Model file for the job. Use its own axes, mm. A direction names the side the tool comes from. Give positions to 0.01 mm unless a question says otherwise; leave off trailing zeros. Write each loop counter-clockwise with the first axis right and the second up, starting at its lowest first coordinate (ties: lowest second). Pieces come first, ordered by that corner, then holes.
```python
from build123d import *

# Parameters (mm, degrees)
SKETCH1_W                                         = 100
SKETCH1_H                                         = 20
BOSS_EXTRUDE1_DEPTH                               = 3
SKETCH2_R                                         = 4
SKETCH2_R_2                                       = 3
SKETCH2_R_3                                       = 5
BOSS_EXTRUDE2_DEPTH                               = 9
CHAMFER1_SIZE                                     = 3
CSK_FOR_6_FLAT_HEAD_MACHINE_SCREW_100_D           = 3.7973
CSK_FOR_6_FLAT_HEAD_MACHINE_SCREW_100_CSINK_D     = 7.0866
CSK_FOR_6_FLAT_HEAD_MACHINE_SCREW_100_CSINK_ANGLE = 100
CSK_FOR_6_FLAT_HEAD_MACHINE_SCREW_2_D             = 3.7973
CSK_FOR_6_FLAT_HEAD_MACHINE_SCREW_2_CSINK_D       = 7.0866
CSK_FOR_6_FLAT_HEAD_MACHINE_SCREW_2_CSINK_ANGLE   = 100
CSK_FOR_6_FLAT_HEAD_MACHINE_SCREW_3_D             = 3.7973
CSK_FOR_6_FLAT_HEAD_MACHINE_SCREW_3_CSINK_D       = 7.0866
CSK_FOR_6_FLAT_HEAD_MACHINE_SCREW_3_CSINK_ANGLE   = 100
CHAMFER2_SIZE                                     = 3
CHAMFER3_SIZE                                     = 3
SKETCH14_R                                        = 3
SKETCH14_R_2                                      = 4
SKETCH14_R_3                                      = 5
BOSS_EXTRUDE3_DEPTH                               = 3
CHAMFER4_SIZE                                     = 3
LPATTERN1_COUNT                                   = 3
LPATTERN1_PITCH                                   = 15
CHAMFER5_SIZE                                     = 7


with BuildPart() as part:
    # Sketch1 → Boss-Extrude1 (new body)
    with BuildSketch(Plane(origin=(0, 0, 0), x_dir=(1, 0, 0), z_dir=(0, 1, 0))):
        Rectangle(SKETCH1_W, SKETCH1_H)
    extrude(amount=BOSS_EXTRUDE1_DEPTH)

    # Sketch2 → Boss-Extrude2 (add)
    with BuildSketch(Plane(origin=(0, 3, 0), x_dir=(1, 0, 0), z_dir=(0, 1, 0))):
        with Locations(Location((-25, 0, 0), (0, 0, 90))):
            Circle(SKETCH2_R)
        with Locations(Location((-40, 0, 0), (0, 0, 90))):
            Circle(SKETCH2_R_2)
        with Locations(Location((-10, 0, 0), (0, 0, 90))):
            Circle(SKETCH2_R_3)
    extrude(amount=BOSS_EXTRUDE2_DEPTH)

    # Chamfer1
    chamfer1_edges = [part.edges().sort_by_distance(p)[0] for p in [
        (-40, 3, 3),
    ]]
    chamfer(chamfer1_edges, length=CHAMFER1_SIZE)

    # CSK for _6 Flat Head Machine Screw _100 (through all)
    with Locations(Plane(origin=(0, 0, 0), x_dir=(-1, 0, 0), z_dir=(0, -1, 0))):
        with Locations((40, 0)):
            CounterSinkHole(CSK_FOR_6_FLAT_HEAD_MACHINE_SCREW_100_D / 2, CSK_FOR_6_FLAT_HEAD_MACHINE_SCREW_100_CSINK_D / 2, counter_sink_angle=CSK_FOR_6_FLAT_HEAD_MACHINE_SCREW_100_CSINK_ANGLE)

    # CSK for _6 Flat Head Machine Screw _ 2 (through all)
    with Locations(Plane(origin=(0, 0, 0), x_dir=(-1, 0, 0), z_dir=(0, -1, 0))):
        with Locations((25, 0)):
            CounterSinkHole(CSK_FOR_6_FLAT_HEAD_MACHINE_SCREW_2_D / 2, CSK_FOR_6_FLAT_HEAD_MACHINE_SCREW_2_CSINK_D / 2, counter_sink_angle=CSK_FOR_6_FLAT_HEAD_MACHINE_SCREW_2_CSINK_ANGLE)

    # CSK for _6 Flat Head Machine Screw _ 3 (through all)
    with Locations(Plane(origin=(0, 0, 0), x_dir=(-1, 0, 0), z_dir=(0, -1, 0))):
        with Locations((10, 0)):
            CounterSinkHole(CSK_FOR_6_FLAT_HEAD_MACHINE_SCREW_3_D / 2, CSK_FOR_6_FLAT_HEAD_MACHINE_SCREW_3_CSINK_D / 2, counter_sink_angle=CSK_FOR_6_FLAT_HEAD_MACHINE_SCREW_3_CSINK_ANGLE)

    # Chamfer2
    chamfer2_edges = [part.edges().sort_by_distance(p)[0] for p in [
        (-25, 3, 4),
    ]]
    chamfer(chamfer2_edges, length=CHAMFER2_SIZE)

    # Chamfer3
    chamfer3_edges = [part.edges().sort_by_distance(p)[0] for p in [
        (-10, 3, 5),
    ]]
    chamfer(chamfer3_edges, length=CHAMFER3_SIZE - 0.0001)  # a hair under: the kernel refuses the full size

    # Sketch14 → Boss-Extrude3 (add)
    with BuildSketch(Plane(origin=(0, 3, 0), x_dir=(1, 0, 0), z_dir=(0, 1, 0))):
        with Locations(Location((10, 0, 0), (0, 0, 90))):
            Circle(SKETCH14_R)
        with Locations(Location((25, 0, 0), (0, 0, 90))):
            Circle(SKETCH14_R_2)
        with Locations(Location((40, 0, 0), (0, 0, 90))):
            Circle(SKETCH14_R_3)
    extrude(amount=BOSS_EXTRUDE3_DEPTH)

    # Chamfer4
    chamfer4_edges = [part.edges().sort_by_distance(p)[0] for p in [
        (10, 3, 3),
        (25, 3, 4),
        (40, 3, 5),
    ]]
    chamfer(chamfer4_edges, length=CHAMFER4_SIZE - 0.0001)  # a hair under: the kernel refuses the full size

    # Sketch18 → CBORE for M3 SBHCS1 (revolve, cut)
    with BuildSketch(Plane(origin=(10, 0, 0), x_dir=(0, 0, -1), z_dir=(1, 0, 0))):
        Polygon((0, 0), (0, 12), (1.8, 12), (1.8, 1.65), (3.35, 1.65), (3.35, 0.025), (3.375, 0), align=None)
    cbore_for_m3_sbhcs1 = revolve(axis=Axis((10, -6.35, 0), (0, 1, 0)), mode=Mode.SUBTRACT)

    # LPattern1: CBORE for M3 SBHCS1 ×3
    with Locations(*[(i * LPATTERN1_PITCH, 0, 0) for i in range(1, LPATTERN1_COUNT)]):
        add(cbore_for_m3_sbhcs1, mode=Mode.SUBTRACT)

    # Chamfer5
    chamfer5_edges = [part.edges().sort_by_distance(p)[0] for p in [
        (50, 1.5, 10),
    ]]
    chamfer(chamfer5_edges, length=CHAMFER5_SIZE)


solid = part.part
```
1. Which spindle directions (+Z, -Z, +X, -X, +Y, -Y) get a long thin tool onto all of the face, cutting with end or side? Do faces 1 (the cylindrical face through (42.97, 0.83, -1.55)), 2 (the flat face through (26, 6, -2)), 3 (the flat face through (-10.1, 12, -2.2)), 4 (the cylindrical face through (-28.966, 8.958, 0.521)), 5 (the cylindrical face through (23.215, 3.795, 0.234)). Say none if no direction does.
Calculated:
face 1: -Y
face 2: +Z, -Z, +X, +Y
face 3: +Z, -Z, +X, -X, +Y
face 4: +Y
face 5: +Y, -Y
2. Probe probe 1 along Z at (x, y) = (25, 0.8); probe 2 along X at (y, z) = (3.5, -5); probe 3 along Y at (x, z) = (-32.5, 3.25). List the from-to ranges inside material, lowest first.
Calculated:
probe 1: z = -10 to -3.35, 3.35 to 10
probe 2: x = -42.29 to -37.71, -29.15 to -20.85, -15.59 to -4.41, 7.71 to 12.29, 20.85 to 29.15, 34.41 to 45.59
probe 3: y = 0 to 3
3. Pull direction X, two halves, no side cores. Call faces 6 (the flat face through (-1, 0, 0)), 7 (the conical face through (13.071, 5.854, 0.682)), 8 (the flat face through (50, 1, -3)): +X half, -X half, draft (parallel to the pull), parting line (faces both ways), or undercut.
Calculated:
face 6: draft
face 7: undercut
face 8: +X half
4. Slice it at B-B, the plane x = -10. Write the cut outline in (y, z), and give its area (3 significant figures).
Calculated:
outline: (0, -10) - (3, -10) - (3, -8) - (6, -5) - (12, -5) - (12, -1.9) - (1.38, -1.9) - (0, -3.54) - close; (0, 3.54) - (1.38, 1.9) - (12, 1.9) - (12, 5) - (6, 5) - (3, 8) - (3, 10) - (0, 10) - close
area: 111 mm2
5. Slice it at D-D, the plane z = 0. State how many separate pieces and enclosed holes the cut face has, and give its area (3 significant figures).
Calculated:
separate pieces: 7
enclosed holes: 0
area: 418 mm2
6. Pin check, flat tips, straight feed: P1, Ø3, axis at x = -25, z = 0, coming from the +Y side; P2, Ø6, axis at x = 25, z = 0, coming from the +Y side; P3, Ø2, axis at x = 26.5, z = -0.5, coming from the -Y side; P4, Ø4, axis at x = -39, y = 9, coming from the +Z side. Stop position of each tip, or through.
Calculated:
P1: passes through
P2: stops at y = 6
P3: stops at y = 1.65
P4: stops at z = 3
7. Slice it at A-A, the plane y = 10. Write the cut outline in (x, z).
Calculated:
outline: circle Ø6 at (-40, 0); circle Ø8 at (-25, 0); circle Ø10 at (-10, 0); hole circle Ø3.8 at (-40, 0); hole circle Ø3.8 at (-25, 0); hole circle Ø3.8 at (-10, 0)
